Geometry: see drawing. Coordinates: mm, zero at the bounding-box minimum. A direction names the side the tool comes from. Coordinates: 2 decimals unless noted, no trailing zeros. Loops run counter-clockwise (first coordinate to the right, second up) from the corner with the lowest first, then second, coordinate; pieces in that order, holes last. Notation, with made-up numbers: (4, 78.5) - (23, 78.5) arc R27 ccw to (23, 99.5) - close; hole circle Ø6 at (54, 53.5). An arc over 180 degrees is marked (long way). Answer in a Markdown table with one row per item.
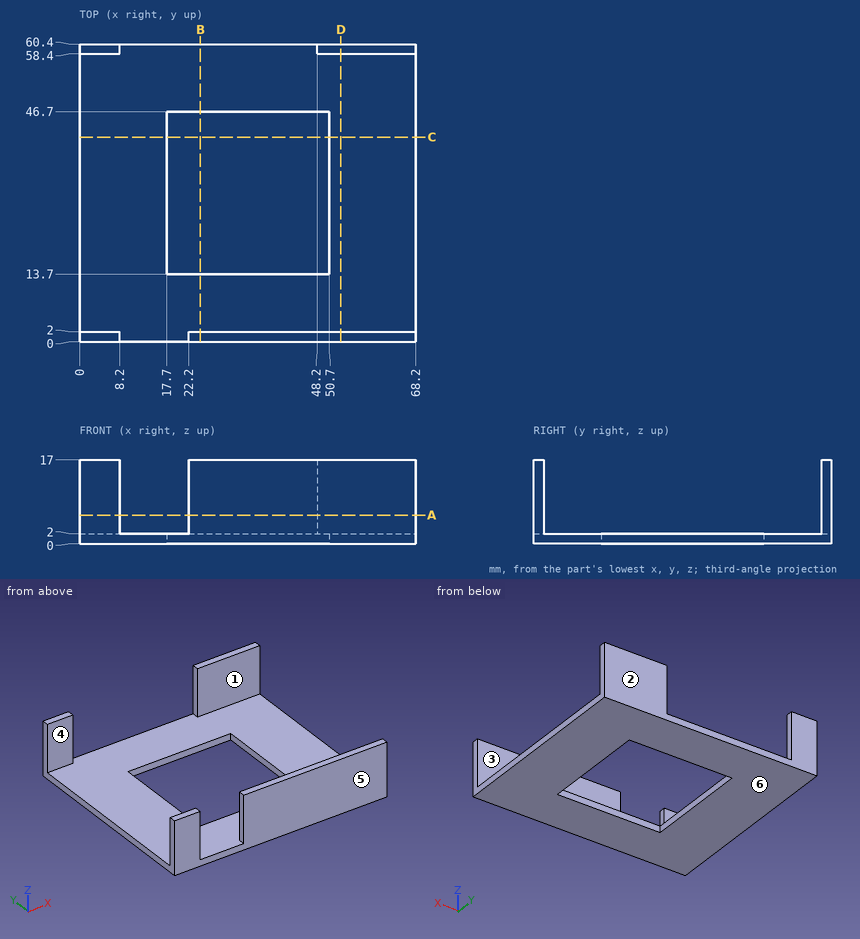
(1) Cut plane B-B on x = 24.5. Output: boundary loops of the cut face in (y, z).
Verdict:
| item | result |
|---|---|
| outline | (0, 0) - (13.7, 0) - (13.7, 2) - (2, 2) - (2, 17) - (0, 17) - close; (46.7, 0) - (60.4, 0) - (60.4, 2) - (46.7, 2) - close |
(2) Cut plane C-C on y = 41.5. Output: boundary loops of the cut face in (x, z).
Verdict:
| item | result |
|---|---|
| outline | (0, 0) - (17.7, 0) - (17.7, 2) - (0, 2) - close; (50.7, 0) - (68.2, 0) - (68.2, 2) - (50.7, 2) - close |
(3) Ray query, probe 1 along Y at (x, z) = (53, 4.75); probe 2 along Z at (x, y) = (7.5, 52.5). Return the intervals inside material, ascending.
Verdict:
| item | result |
|---|---|
| probe 1 | y = 0 to 2, 58.4 to 60.4 |
| probe 2 | z = 0 to 2 |
(4) Pull-direction query (Y, two-part tool) for the marked faces 3, 4, 5 and 6; classes: pulls with the +Y half, pulls with the -Y half, needs draft (parallel to the pull), parting line crosses it, or undercut.
Verdict:
| item | result |
|---|---|
| face 3 | undercut |
| face 4 | undercut |
| face 5 | pulls with the -Y half |
| face 6 | needs draft |
(5) First-contact query: pin 1 Ø5 at (x, z) = (45.5, 6.5) entering from +Y; pin 2 Ø5 at (x, y) = (51.5, 25) entering from +Z. Flat tips, straight axial feed; report the tip coordinate or a pass-through.
Verdict:
| item | result |
|---|---|
| pin 1 | stops at y = 2 |
| pin 2 | stops at z = 2 |
(6) Cut plane A-A on z = 5.75. Output: boundary loops of the cut face in (x, y).
Verdict:
| item | result |
|---|---|
| outline | (0, 0) - (8.2, 0) - (8.2, 2) - (0, 2) - close; (0, 58.4) - (8.2, 58.4) - (8.2, 60.4) - (0, 60.4) - close; (22.2, 0) - (68.2, 0) - (68.2, 2) - (22.2, 2) - close; (48.2, 58.4) - (68.2, 58.4) - (68.2, 60.4) - (48.2, 60.4) - close |
(7) Cut plane D-D on x = 53. Output: boundary loops of the cut face in (y, z), then the cut area to 3 significant figures.
Verdict:
| item | result |
|---|---|
| outline | (0, 0) - (60.4, 0) - (60.4, 17) - (58.4, 17) - (58.4, 2) - (2, 2) - (2, 17) - (0, 17) - close |
| area | 181 mm² |
(8) Access query for the marked faces 1 and 2. Directions: +Z, -Z, +X, -X, +Y, -Y. A direction counts if a zero-diameter tool reaches every point of the face in a straight line with its end or side. Return the directions, or none.
Verdict:
| item | result |
|---|---|
| face 1 | +Z, +X, -X |
| face 2 | +Z, -Z, +X, -X, +Y |
